Work out the finished part from the listing and answer in its coordinate system (mm). Face numbers are marked on the shaded views. A direction names the side the tool comes from. Coordinates: 2 decimals unless noted, no trailing zeros. Loops run counter-clockwise (first coordinate to the right, second up) from the corner with the lowest first, then second, coordinate; pieces in that order, holes last. Notation, with made-up numbers: (10, -21) -> (25, -21) arc R20 cw to (25, 2) -> close; hole circle Ø5 at (61.25, -17). An arc over 180 degrees is marked (long way). One line per question, with ' | ' between items.
```python
from build123d import *

# Parameters (mm, degrees)
F0_W     = 89.748614
F0_H     = 71.432554
F1_DEPTH = 25.4
F2_R     = 18.988019
F3_DEPTH = 25.4
F5_DEPTH = 635


with BuildPart() as f1:
    # F0 (on Top) → F1 (new body)
    with BuildSketch(Plane.XY):
        Rectangle(F0_W, F0_H)
    extrude(amount=F1_DEPTH)

    # F2 (on face) → F3 (join)
    with BuildSketch(Plane.XY.offset(25.4)):
        Circle(F2_R)
    extrude(amount=F3_DEPTH)

    # F4 (on Right) → F5 (cut, symmetric)
    with BuildSketch(Plane.YZ):
        Polygon((-20.643182, 53.957682), (-20.643182, 41.899621), (23.315316, 31.978432), (23.315316, 53.957682), align=None)
    extrude(amount=F5_DEPTH, both=True, mode=Mode.SUBTRACT)


solid = f1.part
```
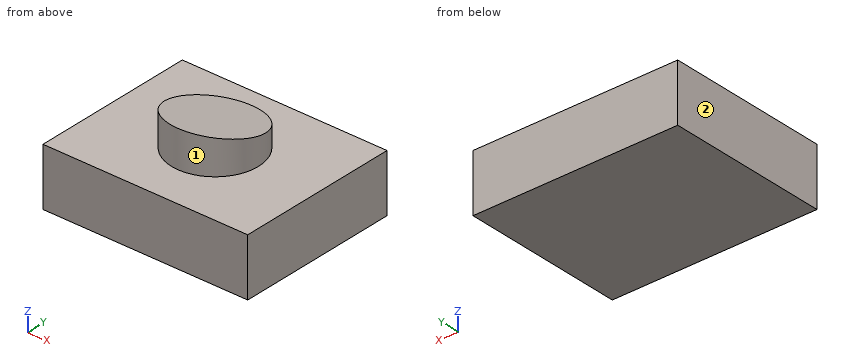
1) Find section D-D (y = 24). Write down the section's boundary in (x, z), plus the area to 3 significant figures.
Check values:
outline: (-44.87, 0) -> (44.87, 0) -> (44.87, 25.4) -> (-44.87, 25.4) -> close | area: 2,280 mm^2
2) Find the intervals of material crossed by line 1 along Z through (x, y) = (15.5, 25.5); line 2 along X through (y, z) = (4, 32.5); line 3 along X through (y, z) = (-14, 39), in increasing order.
Check values:
line 1: z = 0 to 25.4 | line 2: x = -18.56 to 18.56 | line 3: x = -12.83 to 12.83
3) For the marked faces 1 and 2, determine the directions among +Z, -Z, +X, -X, +Y, -Y from which every point of the face is accessible in a straight line to the end or side of a thin tool.
Check values:
face 1: +Z | face 2: +Z, -Z, -X, +Y, -Y
4) Find section A-A (x = 0). Write down the section's boundary in (y, z).
Check values:
outline: (-35.72, 0) -> (35.72, 0) -> (35.72, 25.4) -> (18.99, 25.4) -> (18.99, 32.96) -> (-18.99, 41.53) -> (-18.99, 25.4) -> (-35.72, 25.4) -> close
5) Find section C-C (z = 30). Write down the section's boundary in (x, y).
Check values:
outline: circle Ø37.98 at (0, 0)
6) Flat-ended cylindrical pins translate along their axes: pin 1 (6 mm diameter, centred on x = -35, y = -17.5, fed in from +Z); pin 2 (5 mm diameter, centred on x = -0.5, y = 11, fed in from +Z). Find the tip coordinate at first contact, or state that the pin passes through.
Check values:
pin 1: stops at z = 25.4 | pin 2: stops at z = 35.32
7) Find section B-B (y = 0). Write down the section's boundary in (x, z).
Check values:
outline: (-44.87, 0) -> (44.87, 0) -> (44.87, 25.4) -> (18.99, 25.4) -> (18.99, 37.24) -> (-18.99, 37.24) -> (-18.99, 25.4) -> (-44.87, 25.4) -> close
